```python
from build123d import *

# Parameters (mm, degrees)
BOSS_EXTRUDE1_DEPTH = 6.35
SKETCH2_R           = 3.0988
SKETCH2_W           = 16.51
SKETCH2_H           = 3.175
CUT_EXTRUDE1_DEPTH  = 7.35


with BuildPart() as part:
    # Sketch1 → Boss-Extrude1 (new body)
    with BuildSketch(Plane(origin=(0, 0, 0), x_dir=(1, 0, 0), z_dir=(0, 1, 0))):
        Polygon((-63.5, 0), (-31.75, -54.99261314), (31.75, -54.99261314), (63.5, 0), (31.75, 54.99261314), (-31.75, 54.99261314), align=None)
    extrude(amount=BOSS_EXTRUDE1_DEPTH)

    # Sketch2 → Cut-Extrude1 (cut, through all)
    with BuildSketch(Plane(origin=(0, 6.35, 0), x_dir=(1, 0, 0), z_dir=(0, 1, 0))):
        with Locations((-31.75, -18.330871047)):
            Circle(SKETCH2_R)
        with Locations((0, 36.661742094)):
            Circle(SKETCH2_R)
        with Locations((31.75, -18.330871047)):
            Circle(SKETCH2_R)
        Polygon((-55.290590949, -4.059113577), (-58.040221606, -5.646613577), (-49.785221606, -19.944692993), (-47.035590949, -18.357192993), align=None)
        Polygon((-31.160590949, -45.853499563), (-33.910221606, -47.440999563), (-42.165221606, -33.142920147), (-39.415590949, -31.555420147), align=None)
        Polygon((-31.160590949, 45.853499563), (-33.910221606, 47.440999563), (-42.165221606, 33.142920147), (-39.415590949, 31.555420147), align=None)
        Polygon((-49.785221606, 19.944692993), (-47.035590949, 18.357192993), (-55.290590949, 4.059113577), (-58.040221606, 5.646613577), align=None)
        with Locations((15.875, 51.50011314)):
            Rectangle(SKETCH2_W, SKETCH2_H)
        with Locations((-15.875, 51.50011314)):
            Rectangle(SKETCH2_W, SKETCH2_H)
        Polygon((55.290590949, 4.059113577), (58.040221606, 5.646613577), (49.785221606, 19.944692993), (47.035590949, 18.357192993), align=None)
        Polygon((42.165221606, 33.142920147), (39.415590949, 31.555420147), (31.160590949, 45.853499563), (33.910221606, 47.440999563), align=None)
        Polygon((31.160590949, -45.853499563), (33.910221606, -47.440999563), (42.165221606, -33.142920147), (39.415590949, -31.555420147), align=None)
        Polygon((49.785221606, -19.944692993), (47.035590949, -18.357192993), (55.290590949, -4.059113577), (58.040221606, -5.646613577), align=None)
        with Locations((-15.875, -51.50011314)):
            Rectangle(SKETCH2_W, SKETCH2_H)
        with Locations((15.875, -51.50011314)):
            Rectangle(SKETCH2_W, SKETCH2_H)
    extrude(amount=-CUT_EXTRUDE1_DEPTH, mode=Mode.SUBTRACT)


solid = part.part
```
Here's how the part is built. I have some questions about the finished solid (model axes, mm). Round coordinates to 2 decimals unless told otherwise and drop trailing zeros. Loops run counter-clockwise (first coordinate to the right, second up) from the corner with the lowest first, then second, coordinate; pieces in that order, holes last.
1. Suppose I cut it at D-D, the plane y = 3. Give the number of separate pieces and of enclosed holes in the cut face, and give its area (3 significant figures).
Answers:
separate pieces: 1
enclosed holes: 15
area: 9,760 mm2
2. Thinking about a two-plate mould opening in Z: for faces 1 (the face through (7.62, 3, -51)), 2 (the face through (0, 3, 54.993)), 3 (the face through (0, 3, -54.993)), which applies, released by +Z, released by -Z, zero draft, split by the parting line, or undercut?
Answers:
face 1: undercut
face 2: released by +Z
face 3: released by -Z
3. If I drill on probe 1 along Z at (x, y) = (-22.5, 4); probe 2 along X at (y, z) = (3.25, -12); probe 3 along Z at (x, y) = (31.75, 3.75), over which ranges is the centre line in solid material (lowest first)?
Answers:
probe 1: z = -54.99 to -53.09, -49.91 to 49.91, 53.09 to 54.99
probe 2: x = -56.57 to -54.37, -50.71 to 50.71, 54.37 to 56.57
probe 3: z = -54.99 to -46.19, -44.83 to 15.23, 21.43 to 44.83, 46.19 to 54.99
4. Will these pins go through, and if not, where does the flat tip stop? pin 1 (3 mm diameter, centred on x = -10.5, z = 39.5, fed in from -Y); pin 2 (2.5 mm diameter, centred on y = 3.5, z = -51, fed in from -X); pin 3 (1.5 mm diameter, centred on y = 4, z = -26, fed in from +X); pin 4 (1.6 mm diameter, centred on y = 3, z = 52, fed in from +X).
Answers:
pin 1: stops at y = 0
pin 2: stops at x = -34.78
pin 3: stops at x = 48.92
pin 4: stops at x = 33.94
5. Suppose I cut it at B-B, the plane z = 44. Please give me the cut outline in (x, y).
Answers:
outline: (-38.1, 0) - (-35.9, 0) - (-35.9, 6.35) - (-38.1, 6.35) - close; (-32.23, 0) - (32.23, 0) - (32.23, 6.35) - (-32.23, 6.35) - close; (35.9, 0) - (38.1, 0) - (38.1, 6.35) - (35.9, 6.35) - close
6. Suppose I cut it at C-C, the plane x = 53.5. Please give me the cut outline in (y, z).
Answers:
outline: (0, -17.32) - (6.35, -17.32) - (6.35, -13.51) - (0, -13.51) - close; (0, -7.16) - (6.35, -7.16) - (6.35, 7.16) - (0, 7.16) - close; (0, 13.51) - (6.35, 13.51) - (6.35, 17.32) - (0, 17.32) - close
7. Suppose I cut it at A-A, the plane x = 0. Please give me the cut outline in (y, z).
Answers:
outline: (0, -54.99) - (6.35, -54.99) - (6.35, -39.76) - (0, -39.76) - close; (0, -33.56) - (6.35, -33.56) - (6.35, 54.99) - (0, 54.99) - close
